```python
from build123d import *

# Parameters (mm, degrees)
PAD_DEPTH       = 34
SKETCH_R        = 0.9
POCKET_DEPTH    = 22.001
SKETCH003_W     = 12.8
SKETCH003_H     = 23.2
POCKET001_DEPTH = 22.001
SKETCH005_R     = 1.25
PAD001_DEPTH    = 1.6
SKETCH006_R     = 1.25
PAD002_DEPTH    = 1.6
SKETCH007_W     = 10
SKETCH007_H     = 7
SKETCH007_R     = 0.9
PAD003_DEPTH    = 5.5
CHAMFER_SIZE    = 12
CHAMFER001_SIZE = 1
CHAMFER002_SIZE = 1


with BuildPart() as part:
    # Sketch001 → Pad (new body)
    with BuildSketch(Plane.XZ):
        Polygon((-22, 1.6), (-9, 1.6), (-4, 6.6), (-4, 22.2), (0, 22.2), (0, 6.6), (4, 1.6), (4, 0), (-3.601763, 0), (-22, 0), align=None)
    extrude(amount=PAD_DEPTH)

    # Sketch → Pocket (cut, through all)
    with BuildSketch(Plane(origin=(0, 0, 0), x_dir=(0, 0, 1), z_dir=(1, 0, 0))):
        with Locations((13.4, 30.8)):
            Circle(SKETCH_R)
        with Locations((13.4, 3.6)):
            Circle(SKETCH_R)
    extrude(amount=-POCKET_DEPTH, mode=Mode.SUBTRACT)

    # Sketch003 (on DatumPlane) → Pocket001 (cut, through all)
    with BuildSketch(Plane(origin=(0, 0, 0), x_dir=(0, 0, 1), z_dir=(1, 0, 0))):
        with Locations((13.4, 17.2)):
            Rectangle(SKETCH003_W, SKETCH003_H)
    extrude(amount=-POCKET001_DEPTH, mode=Mode.SUBTRACT)

    # Sketch005 → Pad001 (join)
    with BuildSketch(Plane.XY):
        with BuildLine():
            ThreePointArc((-24.911765, -14.352941), (-26.5, -17), (-24.911765, -19.647059))
            Line((-20.5, -22), (-24.911765, -19.647059))
            Line((-20.5, -12), (-20.5, -22))
            Line((-20.5, -12), (-24.911765, -14.352941))
        make_face()
        with Locations((-23.5, -17)):
            Circle(SKETCH005_R, mode=Mode.SUBTRACT)
    extrude(amount=PAD001_DEPTH)

    # Sketch006 → Pad002 (join)
    with BuildSketch(Plane.XY):
        with BuildLine():
            ThreePointArc((12, -34), (14.963938, -31.463756), (12.916362, -28.143379))
            Line((0, -24), (12.916362, -28.143379))
            Line((0, -34), (0, -24))
            Line((0, -34), (12, -34))
        make_face()
        with Locations((12, -31)):
            Circle(SKETCH006_R, mode=Mode.SUBTRACT)
        with BuildLine():
            ThreePointArc((12.916362, -5.856621), (14.96394, -2.536256), (12.000023, 0))
            Line((0, 0), (12.000023, 0))
            Line((0, 0), (0, -10))
            Line((0, -10), (12.916362, -5.856621))
        make_face()
        with Locations((12, -3)):
            Circle(SKETCH006_R, mode=Mode.SUBTRACT)
    extrude(amount=PAD002_DEPTH)

    # Sketch007 (on Face3 of Pad002) → Pad003 (join)
    with BuildSketch(Plane(origin=(0, 0, 0), x_dir=(0, 0, 1), z_dir=(1, 0, 0))):
        with Locations((13.4, 32.3)):
            Rectangle(SKETCH007_W, SKETCH007_H)
        with Locations((13.4, 30.8)):
            Circle(SKETCH007_R, mode=Mode.SUBTRACT)
        with Locations((13.4, 2.1)):
            Rectangle(SKETCH007_W, SKETCH007_H)
        with Locations((13.4, 3.6)):
            Circle(SKETCH007_R, mode=Mode.SUBTRACT)
    extrude(amount=-PAD003_DEPTH)

    # Chamfer
    chamfer_edges = [part.edges().sort_by_distance(p)[0] for p in [
        (-22, 0, 0.8),
        (-22, -34, 0.8),
    ]]
    chamfer(chamfer_edges, length=CHAMFER_SIZE)

    # Chamfer001
    chamfer001_edges = [part.edges().sort_by_distance(p)[0] for p in [
        (-2, 0, 22.2),
        (-2, -34, 22.2),
    ]]
    chamfer(chamfer001_edges, length=CHAMFER001_SIZE)

    # Chamfer002
    chamfer002_edges = [part.edges().sort_by_distance(p)[0] for p in [
        (-2.75, 1.4, 18.4),
        (-2.75, -35.8, 18.4),
    ]]
    chamfer(chamfer002_edges, length=CHAMFER002_SIZE)


solid = part.part
```
Work out the finished part from the listing and answer in its coordinate system (mm). A direction names the side the tool comes from. Coordinates: 2 decimals unless noted, no trailing zeros. Loops run counter-clockwise (first coordinate to the right, second up) from the corner with the lowest first, then second, coordinate; pieces in that order, holes last. Notation, with made-up numbers: (-0.75, 79) -> (37.25, 79) arc R17 cw to (37.25, 111) -> close; hole circle Ø5 at (60, -10.5). An arc over 180 degrees is marked (long way). Answer as CSV lines item,"result".
Q1. A tool of negligible diameter and unlimited length cuts with its end or side. For faces 1 (the face through (-3, 1.4, 13)), 2 (the face through (0, -17, 21)), 3 (the face through (-2.71, -4.21, 12.74)), 4 (the face through (8.396, -26.693, 0.789)), 5 (the face through (-5.5, -2, 13)), from which of +Z, -Z, +X, -X, +Y, -Y can it reach the whole face along a straight path? Write none if from no direction.
Findings:
face 1,"+Z, -Z, +X, -X, +Y"
face 2,"+Z, +X, +Y, -Y"
face 3,"+X, -X"
face 4,"+Z, -Z, +X"
face 5,"+Z, -X, +Y, -Y"
Q2. Each of these flat-tipped pins is pushed along its axis until it touches: pin 1 (2 mm diameter, centred on y = -31, z = 12.5, fed in from -X); pin 2 (14 mm diameter, centred on x = -14.5, y = -11.5, fed in from +Z); pin 3 (1.4 mm diameter, centred on y = -24, z = 7.5, fed in from -X); pin 4 (1.5 mm diameter, centred on x = 12, y = -3, fed in from +Z). Where does it stop, or does it pass through?
Findings:
pin 1,"stops at x = -5.5"
pin 2,"stops at z = 3.1"
pin 3,"stops at x = -4"
pin 4,"passes through"
Q3. The part is cut by section B-B on z = 7.75. Write down the section's boundary in (x, y), and give its area (3 significant figures).
Findings:
outline,"(-4, -34) -> (0, -34) -> (0, -28.8) -> (-4, -28.8) -> close; (-4, -5.6) -> (0, -5.6) -> (0, 0) -> (-4, 0) -> close"
area,"43.2 mm²"
Q4. The part is cut by section A-A on x = -23.5. Write down the section's boundary in (y, z), and give its area (3 significant figures).
Findings:
outline,"(-20.4, 0) -> (-18.25, 0) -> (-18.25, 1.6) -> (-20.4, 1.6) -> close; (-15.75, 0) -> (-13.6, 0) -> (-13.6, 1.6) -> (-15.75, 1.6) -> close"
area,"6.88 mm²"
Q5. Find the intervals of material crossed by probe 1 along Y at (x, z) = (-2.55, 13.4); probe 2 along Y at (x, z) = (12, 0.4); probe 3 along Z at (x, y) = (-18, -21), in increasing order.
Findings:
probe 1,"y = -35.8 to -31.7, -29.9 to -28.8, -5.6 to -4.5, -2.7 to 1.4"
probe 2,"y = -34 to -32.25, -29.75 to -27.85, -6.15 to -4.25, -1.75 to 0"
probe 3,"z = 0 to 1.6"
Q6. The part is cut by section D-D on y = -19. Write down the section's boundary in (x, z).
Findings:
outline,"(-25.74, 0) -> (4, 0) -> (4, 1.6) -> (0, 6.6) -> (0, 7) -> (-4, 7) -> (-4, 6.6) -> (-9, 1.6) -> (-25.74, 1.6) -> close; (-4, 19.8) -> (0, 19.8) -> (0, 22.2) -> (-4, 22.2) -> close"
Q7. The part is cut by section C-C on y = -3.6. Write down the section's boundary in (x, z), and give its area (3 significant figures).
Findings:
outline,"(-13.6, 0) -> (10.9, 0) -> (10.9, 1.6) -> (4, 1.6) -> (0, 6.6) -> (0, 12.5) -> (-5.5, 12.5) -> (-5.5, 8.4) -> (-4, 8.4) -> (-4, 6.6) -> (-9, 1.6) -> (-13.6, 1.6) -> close; (-5.5, 14.3) -> (0, 14.3) -> (0, 22.2) -> (-4, 22.2) -> (-4, 18.4) -> (-5.5, 18.4) -> close; (13.1, 0) -> (14.94, 0) -> (14.94, 1.6) -> (13.1, 1.6) -> close"
area,"152 mm²"
Q8. For a pull along Z with two mould halves and no side action, classify faces 6 (the face through (-3, -28.8, 13)), 7 (the face through (-23.44, -13.57, 0.79)), 8 (the face through (-6, -17, 0)) as +Z half, -Z half, draft (parallel to the pull), parting line (faces both ways), or undercut.
Findings:
face 6,"undercut"
face 7,"draft"
face 8,"-Z half"
